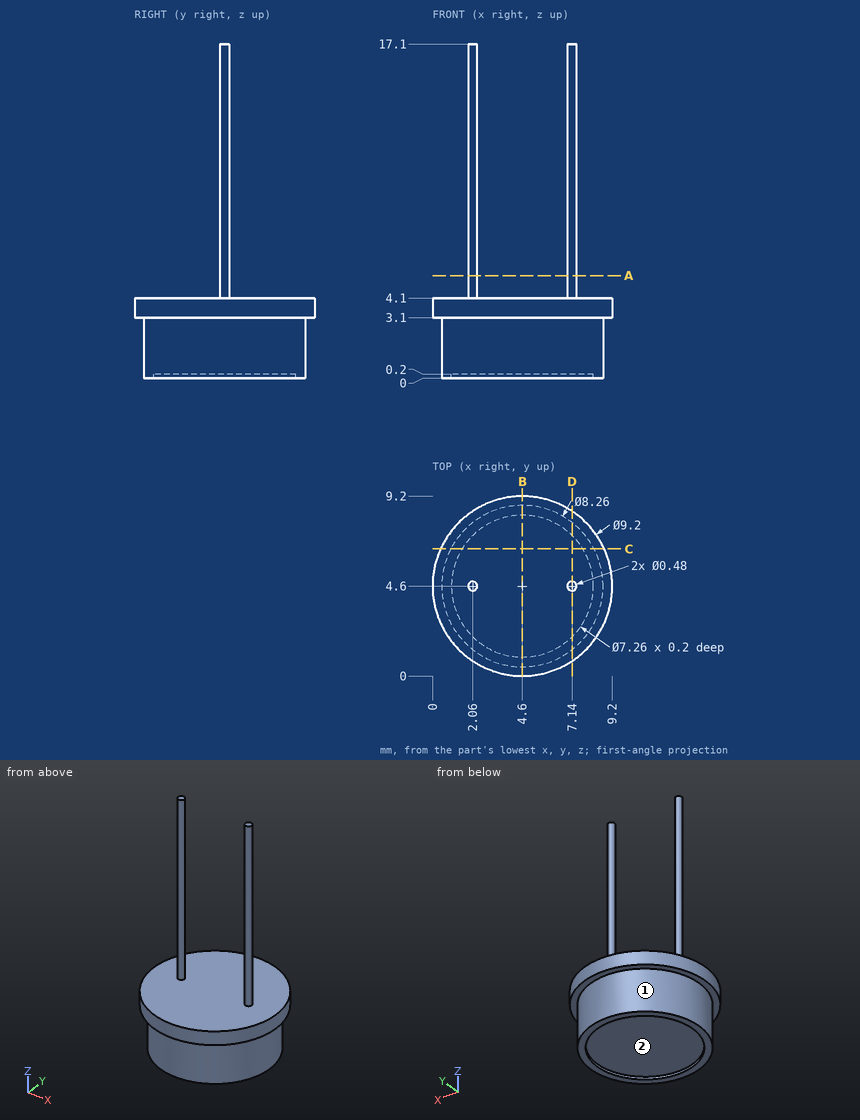
The drawing under review shows one solid part. Ordinate dimensions are in mm from its lowest x, y, z. Round coordinates to 2 decimals unless told otherwise and drop trailing zeros. Order: outer loops, then holes, each group sorted by start corner. A loop starts at its lowest first (then second) coordinate and runs counter-clockwise, first axis right, second up. Notation, with made-up numbers: (-33.5, -36) - (-29.5, -36) arc R27 ccw to (-29.5, 2) - close; hole circle Ø6 at (-38, 5). An arc over 180 degrees is marked (long way). Return JSON: item names as keys, results as strings.
Q1. The part is to be moulded in two halves that separate along X. For the marked faces 1 and 2, say which applies: pulls with the +X half, pulls with the -X half, needs draft (parallel to the pull), parting line crosses it, or undercut.
Computed values:
{"face 1": "parting line crosses it", "face 2": "undercut"}
Q2. Consider section B-B on x = 4.6. Write out the cut boundary in (y, z), plus the area to 3 significant figures.
Computed values:
{"outline": "(0, 3.1) - (0.47, 3.1) - (0.47, 0) - (0.97, 0) - (0.97, 0.2) - (8.23, 0.2) - (8.23, 0) - (8.73, 0) - (8.73, 3.1) - (9.2, 3.1) - (9.2, 4.1) - (0, 4.1) - close", "area": "33.4 mm2"}
Q3. Consider section A-A on z = 5.25. Write out the cut boundary in (x, y), plus the area to 3 significant figures.
Computed values:
{"outline": "circle Ø0.48 at (2.06, 4.6); circle Ø0.48 at (7.14, 4.6)", "area": "0.362 mm2"}
Q4. Consider section D-D on x = 7.14. Write out the cut boundary in (y, z).
Computed values:
{"outline": "(0.76, 3.1) - (1.34, 3.1) - (1.34, 0) - (2.01, 0) - (2.01, 0.2) - (7.19, 0.2) - (7.19, 0) - (7.86, 0) - (7.86, 3.1) - (8.44, 3.1) - (8.44, 4.1) - (4.84, 4.1) - (4.84, 17.1) - (4.36, 17.1) - (4.36, 4.1) - (0.76, 4.1) - close"}
Q5. For pin 1 Ø4 at (y, z) = (1.5, 2.5) entering from -X; pin 2 Ø1 at (x, z) = (3, 4.5) entering from +Y; pin 3 Ø3 at (x, y) = (5.5, 5.5) entering from +Z, all flat-tipped, find the tip position at first contact; note any pin that passes through.
Computed values:
{"pin 1": "stops at x = 0.16", "pin 2": "stops at y = 9.01", "pin 3": "stops at z = 4.1"}
Q6. Consider section C-C on y = 6.5. Write out the cut boundary in (x, z).
Computed values:
{"outline": "(0.41, 3.1) - (0.93, 3.1) - (0.93, 0) - (1.51, 0) - (1.51, 0.2) - (7.69, 0.2) - (7.69, 0) - (8.27, 0) - (8.27, 3.1) - (8.79, 3.1) - (8.79, 4.1) - (0.41, 4.1) - close"}
Q7. Wall thickness on L1, parallel to Y at x = 4.6, z = 0.05; L2, parallel to Z at x = 6.75, y = 4.75; L3, parallel to Z at x = 5.75, y = 1: over which ranges is each line inside the solid? List them lowest first. Write a range as [from, to].
Computed values:
{"L1": "y = [0.47, 0.97], [8.23, 8.73]", "L2": "z = [0.2, 4.1]", "L3": "z = [0, 4.1]"}
